For this review, use the dimensioned drawing (mm, ordinates from the lowest corner) and the shaded views. Coordinates: 2 decimals unless noted, no trailing zeros. Loops run counter-clockwise (first coordinate to the right, second up) from the corner with the lowest first, then second, coordinate; pieces in that order, holes last. Notation, with made-up numbers: M 69.5,83 L 109.5,83 A21 ccw 109.5,101 Z; hole C 74,1 d3. An arc over 180 degrees is marked long. One line per item, written item: value.
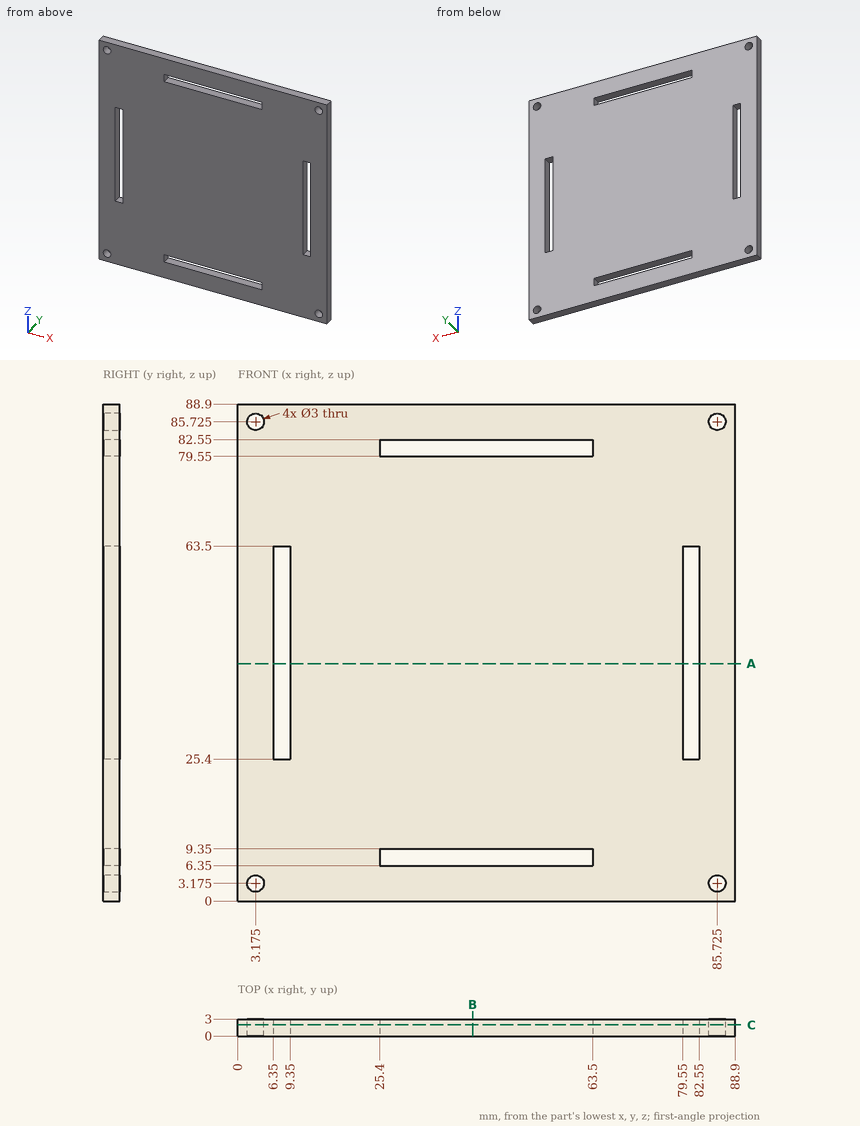
(1) To check wall thickness, follow line 1 along X through (y, z) = (1.75, 61); line 2 along Z through (x, y) = (81, 0.95). State the ranges of each line that lie inside material, in increasing order. Write a range as [from, to].
Reply:
line 1: x = [0, 6.35], [9.35, 79.55], [82.55, 88.9]
line 2: z = [0, 25.4], [63.5, 88.9]
(2) We need section B-B on x = 42. State the section outline as (y, z) points, then the cut area to 3 significant figures.
Reply:
outline: M 0,0 L 3,0 L 3,6.35 L 0,6.35 Z; M 0,9.35 L 3,9.35 L 3,79.55 L 0,79.55 Z; M 0,82.55 L 3,82.55 L 3,88.9 L 0,88.9 Z
area: 249 mm2
(3) We need section C-C on y = 2. State how many separate pieces and enclosed holes the cut face has, then the cut area to 3 significant figures.
Reply:
separate pieces: 1
enclosed holes: 8
area: 7,420 mm2
(4) We need section A-A on z = 42.5. State the section outline as (x, y) points, then the cut area to 3 significant figures.
Reply:
outline: M 0,0 L 6.35,0 L 6.35,3 L 0,3 Z; M 9.35,0 L 79.55,0 L 79.55,3 L 9.35,3 Z; M 82.55,0 L 88.9,0 L 88.9,3 L 82.55,3 Z
area: 249 mm2
